Part model, mm, in its own coordinate system. A direction names the side the tool comes from. Give positions to 0.01 mm unless a question says otherwise; leave off trailing zeros. Order: outer loops, then holes, each group sorted by start corner. A loop starts at its lowest first (then second) coordinate and runs counter-clockwise, first axis right, second up. Notation, with made-up numbers: (22.5, 33.5) - (65.5, 33.5) arc R20 ccw to (65.5, 70.5) - close; hole circle Ø10 at (88.5, 0.5). An arc over 180 degrees is marked (long way). Use a Markdown table: item, result. Add a question column.
from build123d import *

# Parameters (mm, degrees)
F1_DEPTH = 63.5
F0_W     = 25.4
F0_H     = 19.05
F2_DEPTH = 25.4
F3_DEPTH = 7.9375
F5_R     = 6.35


with BuildPart() as f1:
    # F0 (on Front) → F1 (new body, symmetric)
    with BuildSketch(Plane.XZ):
        Polygon((-41.275, -9.525), (41.275, -9.525), (41.275, 9.525), (22.225, 9.525), (-41.275, 9.525), align=None)
    extrude(amount=F1_DEPTH, both=True)

    # F0 (on Front) → F2 (join, symmetric)
    with BuildSketch(Plane.XZ):
        with BuildLine():
            Line((22.225, 9.525), (41.275, 9.525))
            Line((41.275, 9.525), (41.275, 27.0002))
            ThreePointArc((41.275, 27.0002), (45.9246798487, 38.2255201513), (57.15, 42.8752))
            Line((57.15, 42.8752), (60.325, 42.8752))
            Line((60.325, 42.8752), (60.325, 61.9252))
            Line((60.325, 61.9252), (57.15, 61.9252))
            add(Edge.make_bspline(
                [(51.1356519258, 61.403444647), (53.1387058148, 61.5838940905), (55.1443529074, 61.7545470452), (57.15, 61.9252)],
                knots=[0.9452119778, 0.9452119778, 0.9452119778, 0.9452119778, 1, 1, 1, 1], degree=3))
            ThreePointArc((51.1356519258, 61.403444647), (30.4123231049, 49.4691176253), (22.225, 27.0002))
            Line((22.225, 27.0002), (22.225, 9.525))
        make_face()
        with Locations((73.025, 52.4002)):
            Rectangle(F0_W, F0_H)
    extrude(amount=F2_DEPTH, both=True)

    # F0 (on Front) → F3 (join, symmetric)
    with BuildSketch(Plane.XZ):
        with BuildLine():
            add(Edge.make_bspline(
                [(-41.275, 9.525), (-25.9322609375, 26.0151222158), (1.6123086085, 55.6195700492), (35.8274132624, 60.0243688455), (51.1356519258, 61.403444647)],
                knots=[0, 0, 0, 0, 0.5264972724, 0.9452119778, 0.9452119778, 0.9452119778, 0.9452119778], degree=3))
            Line((-41.275, 9.525), (22.225, 9.525))
            Line((22.225, 9.525), (22.225, 27.0002))
            ThreePointArc((22.225, 27.0002), (30.4123231049, 49.4691176253), (51.1356519258, 61.403444647))
        make_face()
    extrude(amount=F3_DEPTH, both=True)

    # F0 (on Front) → F4 (revolve)
    with BuildSketch(Plane.XZ):
        Polygon((85.725, 61.9252), (85.725, 42.8752), (85.725, 38.1), (111.125, 38.1), (111.125, 66.675), (85.725, 66.675), align=None)
    revolve(axis=Axis((85.725, 0, 52.3875), (0, 0, 1)))

    # F5
    f5_edges = [f1.edges().sort_by_distance(p)[0] for p in [
        (41.275, -63.5, 0),
        (-41.275, -63.5, 0),
        (41.275, 63.5, 0),
        (-41.275, 63.5, 0),
    ]]
    fillet(f5_edges, radius=F5_R)


solid = f1.part
1. Cut at A-A (z = -3). Write the cut outline in (x, y) (3 decimals).
2. Mould opens along X. For faces 5 (the face through (30.633, 16.547, 49.73)), 6 (the face through (86, 0, 38.1)), 7 (the face through (45.8, -0.4, 38.1)), 8 (the face through (60, 2, 42.875)) say: released by +X, released by -X, zero draft, split by the parting line, or undercut.
3. Cut at B-B (x = 65). Write the cut outline in (y, z) (1 decimal).
4. Cut at C-C (y = 30). Write the cut outline in (x, z) (3 decimals).
5. Pin check, flat tips, straight feed: P1, Ø5, axis at x = 21, y = -35.5, coming from the +Z side (3 decimals); P2, Ø10, axis at x = -23.5, z = 38.5, coming from the +Y side; P3, Ø23, axis at x = 78, y = 8, coming from the -Z side; P4, Ø15.5, axis at x = 20, z = 31, coming from the +Y side. Stop position of each tip, or through.
6. Tool access for faces 1 (the face through (39.464, -61.59, 0.133)), 2 (the face through (41.275, -1, 4)), 3 (the face through (6, -7.938, 30)), 4 (the face through (22.225, 17, 18)): list every direction of +Z, -Z, +X, -X, +Y, -Y with a clear straight run to the whole face (end or side of a thin tool).
7. Drill centre lines: probe 1 along X at (y, z) = (46.5, 8.5) (3 decimals); probe 2 along Z at (x, y) = (-22.5, -51.5) (3 decimals); probe 3 along Y at (x, z) = (28.5, 32.5). Where is each one in solid material? Low to high. Write a range as [from, to].
Responses:
| question | item | result |
|---|---|---|
| 1 | outline | (-41.275, -57.15) arc R6.35 ccw to (-34.925, -63.5) - (34.925, -63.5) arc R6.35 ccw to (41.275, -57.15) - (41.275, 57.15) arc R6.35 ccw to (34.925, 63.5) - (-34.925, 63.5) arc R6.35 ccw to (-41.275, 57.15) - close |
| 2 | face 5 | released by -X |
| 2 | face 6 | zero draft |
| 2 | face 7 | undercut |
| 2 | face 8 | undercut |
| 3 | outline | (-25.4, 42.9) - (-14.7, 42.9) - (-14.7, 38.1) - (14.7, 38.1) - (14.7, 42.9) - (25.4, 42.9) - (25.4, 61.9) - (14.7, 61.9) - (14.7, 66.7) - (-14.7, 66.7) - (-14.7, 61.9) - (-25.4, 61.9) - close |
| 4 | outline | (-41.275, -9.525) - (41.275, -9.525) - (41.275, 9.525) - (-41.275, 9.525) - close |
| 5 | P1 | stops at z = 9.525 |
| 5 | P2 | passes through |
| 5 | P3 | stops at z = 38.1 |
| 5 | P4 | stops at y = 25.4 |
| 6 | face 1 | +Z, -Z, +X, -Y |
| 6 | face 2 | -Z, +X, +Y, -Y |
| 6 | face 3 | +Z, -X, -Y |
| 6 | face 4 | +Z, -X, +Y |
| 7 | probe 1 | x = [-41.275, 41.275] |
| 7 | probe 2 | z = [-9.525, 9.525] |
| 7 | probe 3 | y = [-25.4, 25.4] |
